Could you check a few things on this model? Use its own coordinates, in mm. Coordinates: 2 decimals unless noted, no trailing zeros. Write each loop counter-clockwise with the first axis right and the second up, starting at its lowest first coordinate (ties: lowest second). Pieces come first, ordered by that corner, then holes.
Item 1: I want a section at A-A on z = 56. Please give me the cut outline in (x, y).
Item 2: If I drill on probe 1 along Z at (x, y) = (9.5, 1.5); probe 2 along Y at (x, z) = (3.5, -136); probe 3 along Y at (x, z) = (2, 47.5), over which ranges is the centre line in solid material (lowest first)?
Item 3: I want a section at B-B on x = 8. State how many separate pieces and enclosed holes the cut face has, then the cut area to 3 significant figures.
Item 4: For P1, Ø5, axis at x = 5, z = 156.5, coming from the -Y side; P2, Ø6, axis at x = 1, y = 231.5, coming from the +Z side, each with a flat end and sliding along its axis, tell me the tip position at first contact or that it passes through.
from build123d import *

# Parameters (mm, degrees)
BOSS_EXTRUDE1_DEPTH   = 10.16
SKETCH2_W             = 76.2
SKETCH2_H             = 10.16
CUT_EXTRUDE1_DEPTH    = 4.572
CHAMFER1_SIZE         = 38.1
CHAMFER1_SIZE2        = 65.991135768
CHAMFER1_PART_2_SIZE  = 38.1
CHAMFER1_PART_2_SIZE2 = 65.991135768
FILLET1_R             = 25.4
CUT_EXTRUDE2_DEPTH    = 26.416


with BuildPart() as part:
    # Sketch1 → Boss-Extrude1 (new body)
    with BuildSketch(Plane(origin=(0, 0, 0), x_dir=(0, 0, -1), z_dir=(1, 0, 0))):
        Polygon((-203.2, 0), (-203.2, 254), (-203.2, 279.4), (203.2, 279.4), (203.2, 254), (203.2, 0), (203.2, -76.2), (-203.2, -76.2), align=None)
        with BuildLine():
            Line((-95.25, 234.95), (95.25, 234.95))
            ThreePointArc((95.25, 234.95), (114.3, 215.9), (95.25, 196.85))
            Line((95.25, 196.85), (-95.25, 196.85))
            ThreePointArc((-95.25, 196.85), (-114.3, 215.9), (-95.25, 234.95))
        make_face(mode=Mode.SUBTRACT)
    extrude(amount=BOSS_EXTRUDE1_DEPTH)

    # Sketch2 → Cut-Extrude1 (cut)
    with BuildSketch(Plane(origin=(0, 0, 0), x_dir=(0, 0, -1), z_dir=(1, 0, 0))):
        with Locations((-158.75, 127)):
            Rectangle(SKETCH2_W, SKETCH2_H)
        with Locations((0, 127)):
            Rectangle(SKETCH2_W, SKETCH2_H)
        with Locations((158.75, 127)):
            Rectangle(SKETCH2_W, SKETCH2_H)
    extrude(amount=CUT_EXTRUDE1_DEPTH, mode=Mode.SUBTRACT)

    # Chamfer1
    chamfer1_edges = [part.edges().sort_by_distance(p)[0] for p in [
        (5.08, 279.4, 203.2),
        (5.08, 279.4, -203.2),
    ]]
    chamfer1_side = [part.faces().sort_by_distance(p)[0] for p in [
        (5.08, 279.4, 0),
    ]]
    chamfer(chamfer1_edges, length=CHAMFER1_SIZE, length2=CHAMFER1_SIZE2, reference=chamfer1_side[0])

    # Chamfer1 part 2
    chamfer1_part_2_edges = [part.edges().sort_by_distance(p)[0] for p in [
        (5.08, -76.2, -203.2),
        (5.08, -76.2, 203.2),
    ]]
    chamfer1_part_2_side = [part.faces().sort_by_distance(p)[0] for p in [
        (5.08, -76.2, 0),
    ]]
    chamfer(chamfer1_part_2_edges, length=CHAMFER1_PART_2_SIZE, length2=CHAMFER1_PART_2_SIZE2, reference=chamfer1_part_2_side[0])

    # Fillet1
    fillet1_edges = [part.edges().sort_by_distance(p)[0] for p in [
        (5.08, 213.408864232, -203.2),
        (5.08, -10.208864232, -203.2),
        (5.08, -76.2, 165.1),
        (5.08, -76.2, -165.1),
        (5.08, 213.408864232, 203.2),
        (5.08, -10.208864232, 203.2),
        (5.08, 279.4, -165.1),
        (5.08, 279.4, 165.1),
    ]]
    fillet(fillet1_edges, radius=FILLET1_R)

    # Sketch4 → Cut-Extrude2 (cut)
    with BuildSketch(Plane(origin=(0, 0, 0), x_dir=(0, 0, -1), z_dir=(1, 0, 0))):
        with BuildLine():
            Line((-171.45, 102.87), (-120.65, 102.87))
            ThreePointArc((-120.65, 102.87), (-116.159871939, 101.010128061), (-114.3, 96.52))
            Line((-114.3, 96.52), (-114.3, -17.78))
            ThreePointArc((-114.3, -17.78), (-116.159871939, -22.270128061), (-120.65, -24.13))
            Line((-120.65, -24.13), (-171.45, -24.13))
            ThreePointArc((-171.45, -24.13), (-175.940128061, -22.270128061), (-177.8, -17.78))
            Line((-177.8, -17.78), (-177.8, 96.52))
            ThreePointArc((-177.8, 96.52), (-175.940128061, 101.010128061), (-171.45, 102.87))
        make_face()
        with BuildLine():
            Line((-76.2, 115.57), (-25.4, 115.57))
            ThreePointArc((-25.4, 115.57), (-20.909871939, 113.710128061), (-19.05, 109.22))
            Line((-19.05, 109.22), (-19.05, -30.48))
            ThreePointArc((-19.05, -30.48), (-20.909871939, -34.970128061), (-25.4, -36.83))
            Line((-25.4, -36.83), (-76.2, -36.83))
            ThreePointArc((-76.2, -36.83), (-80.690128061, -34.970128061), (-82.55, -30.48))
            Line((-82.55, -30.48), (-82.55, 109.22))
            ThreePointArc((-82.55, 109.22), (-80.690128061, 113.710128061), (-76.2, 115.57))
        make_face()
        with BuildLine():
            Line((19.05, 109.22), (19.05, -30.48))
            ThreePointArc((19.05, -30.48), (20.909871939, -34.970128061), (25.4, -36.83))
            Line((25.4, -36.83), (76.2, -36.83))
            ThreePointArc((76.2, -36.83), (80.690128061, -34.970128061), (82.55, -30.48))
            Line((82.55, -30.48), (82.55, 109.22))
            ThreePointArc((82.55, 109.22), (80.690128061, 113.710128061), (76.2, 115.57))
            Line((76.2, 115.57), (25.4, 115.57))
            ThreePointArc((25.4, 115.57), (20.909871939, 113.710128061), (19.05, 109.22))
        make_face()
        with BuildLine():
            Line((114.3, 96.52), (114.3, -17.78))
            ThreePointArc((114.3, -17.78), (116.159871939, -22.270128061), (120.65, -24.13))
            Line((120.65, -24.13), (171.45, -24.13))
            ThreePointArc((171.45, -24.13), (175.940128061, -22.270128061), (177.8, -17.78))
            Line((177.8, -17.78), (177.8, 96.52))
            ThreePointArc((177.8, 96.52), (175.940128061, 101.010128061), (171.45, 102.87))
            Line((171.45, 102.87), (120.65, 102.87))
            ThreePointArc((120.65, 102.87), (116.159871939, 101.010128061), (114.3, 96.52))
        make_face()
    extrude(amount=CUT_EXTRUDE2_DEPTH, mode=Mode.SUBTRACT)


solid = part.part
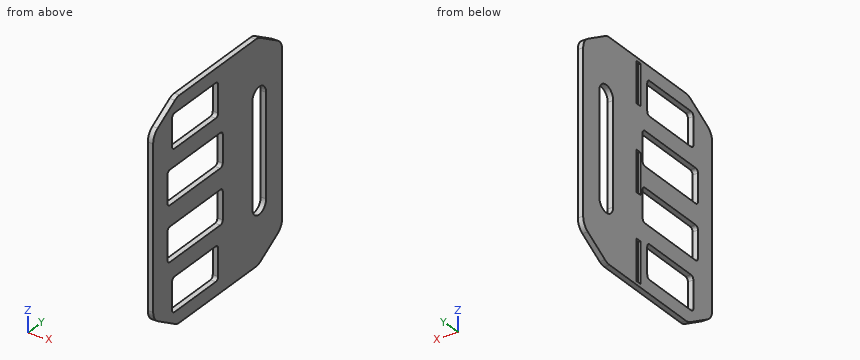
Response values:
1. outline: (0, -76.2) - (10.16, -76.2) - (10.16, -36.83) - (0, -36.83) - close; (0, 115.57) - (10.16, 115.57) - (10.16, 196.85) - (0, 196.85) - close; (0, 234.95) - (10.16, 234.95) - (10.16, 279.4) - (0, 279.4) - close
2. probe 1: z = -203.2 to -177.8, -114.3 to -82.55, -19.05 to 19.05, 82.55 to 114.3, 177.8 to 203.2
2. probe 2: y = -76.2 to -24.13, 102.87 to 121.92, 132.08 to 279.4
2. probe 3: y = -76.2 to -36.83, 115.57 to 196.85, 234.95 to 279.4
3. separate pieces: 1
3. enclosed holes: 5
3. area: 95,600 mm2
4. P1: stops at y = -75.95
4. P2: stops at z = 194.49
